Verification items for the finished model (mm, model axes). Face numbers are marked on the shaded views. A direction names the side the tool comes from. Give positions to 0.01 mm unless a question says otherwise; leave off trailing zeros. Loops run counter-clockwise (first coordinate to the right, second up) from the corner with the lowest first, then second, coordinate; pieces in that order, holes last. Notation, with made-up numbers: (-27.75, 68) - (8.25, 68) arc R19 ccw to (8.25, 75) - close; hole circle Ø2 at (39, 35.5). An arc over 180 degrees is marked (long way). Use one line per item in the form item = value.
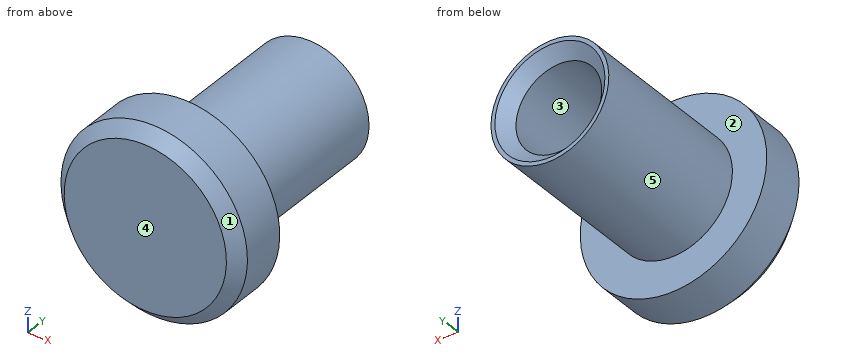
```python
from build123d import *

# Parameters (mm, degrees)
F2_SIZE = 0.8255


with BuildPart() as f1:
    # F0 (on Right) → F1 (revolve)
    with BuildSketch(Plane.YZ):
        Polygon((0, 6.35), (0, 0), (2.689886, 0), (4.445, 2.921), (15.24, 2.921), (15.24, 4.0132), (3.81, 4.0132), (3.81, 6.35), align=None)
    revolve(axis=Axis((0, 1.344943, 0), (0, -1, 0)))

    # F2
    f2_edges = [f1.edges().sort_by_distance(p)[0] for p in [
        (0, 15.24, -2.921),
        (0, 0, -6.35),
    ]]
    chamfer(f2_edges, length=F2_SIZE)


solid = f1.part
```
1. Depth check by flat-ended pin: pin 1 Ø1.5 at (x, y) = (3, 11.5) entering from +Z; pin 2 Ø4 at (x, y) = (-2, 7) entering from -Z; pin 3 Ø1.5 at (x, y) = (-1, 12.5) entering from +Z. Enter the tip coordinate at first touch or a pass-through.
Result set:
pin_1 = 3.32
pin_2 = -4.01
pin_3 = 4.01
2. Section check A-A, the plane y = 7.5. Record the cut outline in (x, z), then the cut area to 3 significant figures.
Result set:
outline = circle Ø8.03 at (0, 0); hole circle Ø5.84 at (0, 0)
area = 23.8 mm²
3. Draft check along X on the marked faces 3, 4 and 5. Enter one of: released by +X, released by -X, zero draft, split by the parting line, or undercut.
Result set:
face_3 = undercut
face_4 = zero draft
face_5 = split by the parting line
4. Scan lines: probe 1 along Z at (x, y) = (0, 11); probe 2 along Z at (x, y) = (1, 7.25). Record each from-to range of solid material in increasing order.
Result set:
probe_1 = -4.01 to -2.92, 2.92 to 4.01
probe_2 = -3.89 to -2.74, 2.74 to 3.89
5. Tool access check on the marked faces 1 and 2. Record the directions out of +Z, -Z, +X, -X, +Y, -Y that give a thin tool (end or side, any length) a straight path to the whole face; none if there is none.
Result set:
face_1 = -Y
face_2 = +Y
